Work out the finished part from the listing and answer in its coordinate system (mm). A direction names the side the tool comes from. Give positions to 0.01 mm unless a question says otherwise; leave off trailing zeros. Order: outer loops, then holes, each group sorted by start corner. A loop starts at its lowest first (then second) coordinate and runs counter-clockwise, first axis right, second up.
```python
from build123d import *

# Parameters (mm, degrees)
F0_R     = 10.873019
F1_DEPTH = 5.08


with BuildPart() as f1:
    # F0 (on Front) → F1 (new body)
    with BuildSketch(Plane.XZ):
        with BuildLine():
            ThreePointArc((-7.49769, -22.859156), (-3.613745, -29.461579), (0, -36.215678))
            ThreePointArc((0, -36.215678), (3.613745, -29.461579), (7.49769, -22.859156))
            ThreePointArc((7.49769, -22.859156), (20.904776, -17.20558), (34.945954, -21.021102))
            ThreePointArc((34.945954, -21.021102), (38.568356, -29.052358), (41.93056, -37.195973))
            ThreePointArc((41.93056, -37.195973), (45.206649, -29.069506), (48.670087, -21.021102))
            ThreePointArc((48.670087, -21.021102), (49.842619, -25.920576), (50.998289, -30.824054))
            ThreePointArc((50.998289, -30.824054), (54.439372, -25.929613), (57.860356, -21.021102))
            ThreePointArc((57.860356, -21.021102), (62.956488, 0), (57.860356, 21.021102))
            ThreePointArc((57.860356, 21.021102), (54.439372, 25.929613), (50.998289, 30.824054))
            ThreePointArc((50.998289, 30.824054), (49.842619, 25.920576), (48.670087, 21.021102))
            ThreePointArc((48.670087, 21.021102), (45.206649, 29.069506), (41.93056, 37.195973))
            ThreePointArc((41.93056, 37.195973), (38.568356, 29.052358), (34.945954, 21.021102))
            ThreePointArc((34.945954, 21.021102), (20.904776, 17.20558), (7.49769, 22.859156))
            Line((7.49769, 22.859156), (7.49769, 39.19407))
            Line((7.49769, 39.19407), (2.909613, 27.099166))
            ThreePointArc((2.909613, 27.099166), (0.068039, 28.124589), (-2.773535, 27.099166))
            Line((-2.773535, 27.099166), (-7.49769, 39.19407))
            ThreePointArc((-7.49769, 39.19407), (-7.397431, 31.026613), (-7.49769, 22.859156))
            ThreePointArc((-7.49769, 22.859156), (-20.904776, 17.20558), (-34.945954, 21.021102))
            ThreePointArc((-34.945954, 21.021102), (-38.568356, 29.052358), (-41.93056, 37.195973))
            ThreePointArc((-41.93056, 37.195973), (-45.206649, 29.069506), (-48.670087, 21.021102))
            ThreePointArc((-48.670087, 21.021102), (-49.842619, 25.920576), (-50.998289, 30.824054))
            ThreePointArc((-50.998289, 30.824054), (-54.439372, 25.929613), (-57.860356, 21.021102))
            ThreePointArc((-57.860356, 21.021102), (-62.956488, 0), (-57.860356, -21.021102))
            ThreePointArc((-57.860356, -21.021102), (-54.439372, -25.929613), (-50.998289, -30.824054))
            ThreePointArc((-50.998289, -30.824054), (-49.842619, -25.920576), (-48.670087, -21.021102))
            ThreePointArc((-48.670087, -21.021102), (-45.206649, -29.069506), (-41.93056, -37.195973))
            ThreePointArc((-41.93056, -37.195973), (-38.568356, -29.052358), (-34.945954, -21.021102))
            ThreePointArc((-34.945954, -21.021102), (-20.904776, -17.20558), (-7.49769, -22.859156))
        make_face()
        Polygon((-47.67337, 9.656313), (-36.52322, 9.656313), (-30.948145, 0), (-36.52322, -9.656313), (-47.67337, -9.656313), (-53.248445, 0), align=None, mode=Mode.SUBTRACT)
        Circle(F0_R, mode=Mode.SUBTRACT)
        Polygon((30.948145, 0), (36.52322, 9.656313), (47.67337, 9.656313), (53.248445, 0), (47.67337, -9.656313), (36.52322, -9.656313), align=None, mode=Mode.SUBTRACT)
    extrude(amount=F1_DEPTH)


solid = f1.part
```
1. Given P1, Ø3, axis at x = -15.5, y = -2.5, coming from the +Z side; P2, Ø2, axis at y = -3.5, z = -7.5, coming from the -X side; P3, Ø3, axis at x = -32.5, y = -1.5, coming from the -Z side, each flat-ended and moving along its own axis, determine where each tip first touches the part or whether it passes through.
Findings below:
P1: stops at z = 18.8
P2: stops at x = -62.49
P3: stops at z = -20.41
2. The part is cut by section B-B (z = -28.5). Write down the section's boundary in (x, y).
Findings below:
outline: (-52.64, -5.08) - (-50.45, -5.08) - (-50.45, 0) - (-52.64, 0) - close; (-45.44, -5.08) - (-38.33, -5.08) - (-38.33, 0) - (-45.44, 0) - close; (-4.16, -5.08) - (4.16, -5.08) - (4.16, 0) - (-4.16, 0) - close; (38.33, -5.08) - (45.44, -5.08) - (45.44, 0) - (38.33, 0) - close; (50.45, -5.08) - (52.64, -5.08) - (52.64, 0) - (50.45, 0) - close
3. Which of the six approach directions +Z, -Z, +X, -X, +Y, -Y give full straight-line access (tool end or side, diameter ignored) to faces 5 (the face through (3.56, -2.5, -29.56)), 6 (the face through (-5.1, -2.5, 33.06)), 7 (the face through (-54.49, -2.5, -25.86)), 8 (the face through (-50.42, -2.5, -4.9))?
Findings below:
face 5: -Z, +Y, -Y
face 6: +Z, +Y, -Y
face 7: -Z, -X, +Y, -Y
face 8: +Y, -Y
4. The part is cut by section D-D (y = -4.25). State how many separate pieces and enclosed holes the cut face has, then the cut area to 3 significant figures.
Findings below:
separate pieces: 1
enclosed holes: 3
area: 4,770 mm2
5. The mould has two halves that part along Z. Classify faces 1 (the face through (5.845, -2.504, 9.168)), 2 (the face through (5.236, -2.504, 33.231)), 3 (the face through (13, 0, 2)), 4 (the face through (-38.62, -2.5, -29.17)): pulls with the +Z half, pulls with the -Z half, needs draft (parallel to the pull), parting line crosses it, or undercut.
Findings below:
face 1: undercut
face 2: pulls with the +Z half
face 3: needs draft
face 4: pulls with the -Z half
6. The part is cut by section A-A (z = -3). Write down the section's boundary in (x, y).
Findings below:
outline: (-62.86, -5.08) - (-51.52, -5.08) - (-51.52, 0) - (-62.86, 0) - close; (-32.68, -5.08) - (-10.45, -5.08) - (-10.45, 0) - (-32.68, 0) - close; (10.45, -5.08) - (32.68, -5.08) - (32.68, 0) - (10.45, 0) - close; (51.52, -5.08) - (62.86, -5.08) - (62.86, 0) - (51.52, 0) - close
7. Straight lines are drawn through the part: probe 1 along X at (y, z) = (-3.45, 27); probe 2 along X at (y, z) = (-0.5, -27); probe 3 along X at (y, z) = (-4.3, -9.5). For each, find the intervals that lie inside material, in ascending order.
Findings below:
probe 1: x = -53.69 to -50.1, -46.08 to -37.67, -7.42 to 7.5, 37.67 to 46.08, 50.1 to 53.69
probe 2: x = -53.69 to -50.1, -46.08 to -37.67, -5.02 to 5.02, 37.67 to 46.08, 50.1 to 53.69
probe 3: x = -61.96 to -47.76, -36.43 to -5.29, 5.29 to 36.43, 47.76 to 61.96
8. The part is cut by section C-C (x = -32.5). Write down the section's boundary in (y, z), then the cut area to 3 significant figures.
Findings below:
outline: (-5.08, -19.58) - (0, -19.58) - (0, -2.69) - (-5.08, -2.69) - close; (-5.08, 2.69) - (0, 2.69) - (0, 19.58) - (-5.08, 19.58) - close
area: 172 mm2
